```python
from build123d import *

# Parameters (mm, degrees)
CROQUIS1_W              = 35.7
CROQUIS1_H              = 4
CROQUIS1_R              = 1
SALIENTE_EXTRUIR1_DEPTH = 2.2
REDONDEO1_R             = 2


with BuildPart() as part:
    # Croquis1 → Saliente-Extruir1 (new body)
    with BuildSketch(Plane.XY):
        with Locations((-44.497764467, 10.416666667)):
            Rectangle(CROQUIS1_W, CROQUIS1_H)
        with Locations((-59.847764467, 10.416666667)):
            Circle(CROQUIS1_R, mode=Mode.SUBTRACT)
        with Locations((-29.147764467, 10.416666667)):
            Circle(CROQUIS1_R, mode=Mode.SUBTRACT)
    extrude(amount=SALIENTE_EXTRUIR1_DEPTH)

    # Redondeo1
    redondeo1_edges = [part.edges().sort_by_distance(p)[0] for p in [
        (-62.347764467, 8.416666667, 1.1),
        (-62.347764467, 12.416666667, 1.1),
        (-26.647764467, 8.416666667, 1.1),
        (-26.647764467, 12.416666667, 1.1),
    ]]
    fillet(redondeo1_edges, radius=REDONDEO1_R - 0.0001)  # a hair under: the kernel refuses the full size


solid = part.part
```
Verification items for the finished model (mm, model axes). Give positions to 0.01 mm unless a question says otherwise; leave off trailing zeros. Order: outer loops, then holes, each group sorted by start corner. A loop starts at its lowest first (then second) coordinate and runs counter-clockwise, first axis right, second up. Notation, with made-up numbers: (-34, -37.5) - (19, -37.5) arc R35 ccw to (19, -0.5) - close; hole circle Ø3 at (45.25, 67.25). An arc over 180 degrees is marked (long way). Answer as CSV lines item,"result". Start each with the question number.
Item 1: Mould release check, pull along Y, two halves, no side actions. Record for faces 1 (the face through (-45, 10, 2.2)), 2 (the face through (-45, 12.417, 1)), 3 (the face through (-28.224, 10.034, 1.085)): released by +Y, released by -Y, zero draft, split by the parting line, or undercut.
Item 2: Section check A-A, the plane x = -60. Record the boundary of the cut face in (y, z).
Item 3: Section check B-B, the plane z = 1.7. State how many separate pieces and enclosed holes the cut face has, plus the area to 3 significant figures.
Item 4: Section check C-C, the plane y = 9.85. Record the boundary of the cut face in (x, z), plus the area to 3 significant figures.
Item 5: Section check D-D, the plane x = -29.5. Record the boundary of the cut face in (y, z).
Item 6: Material ranges on L1, parallel to X at y = 11.3, z = 0.5; L2, parallel to X at y = 9.75, z = 1.65; L3, parallel to Y at x = -60, z = 2, recorded low to high.
Item 7: Gauge pin test, flat ends, axial feed: pin 1 (1.6 mm diameter, centred on x = -59.85, y = 10.42, fed in from -Z); pin 2 (2 mm diameter, centred on x = -47.5, y = 11.5, fed in from -Z). Record the tip position at first contact, or that the pin passes through.
Filled in:
1,face 1,"zero draft"
1,face 2,"released by +Y"
1,face 3,"undercut"
2,outline,"(8.42, 0) - (9.43, 0) - (9.43, 2.2) - (8.42, 2.2) - close; (11.41, 0) - (12.42, 0) - (12.42, 2.2) - (11.41, 2.2) - close"
3,separate pieces,"1"
3,enclosed holes,"2"
3,area,"133 mm^2"
4,outline,"(-62.27, 0) - (-60.67, 0) - (-60.67, 2.2) - (-62.27, 2.2) - close; (-59.02, 0) - (-29.97, 0) - (-29.97, 2.2) - (-59.02, 2.2) - close; (-28.32, 0) - (-26.73, 0) - (-26.73, 2.2) - (-28.32, 2.2) - close"
4,area,"70.9 mm^2"
5,outline,"(8.42, 0) - (9.48, 0) - (9.48, 2.2) - (8.42, 2.2) - close; (11.35, 0) - (12.42, 0) - (12.42, 2.2) - (11.35, 2.2) - close"
6,L1,"-62.14 to -60.32, -59.38 to -29.62, -28.68 to -26.85"
6,L2,"-62.23 to -60.59, -59.1 to -29.89, -28.4 to -26.76"
6,L3,"8.42 to 9.43, 11.41 to 12.42"
7,pin 1,"through"
7,pin 2,"z = 0"
